Design review of the part built by this model. Coordinates are the model's own, in mm. Face numbers are marked on the shaded views. A direction names the side the tool comes from. Coordinates: 2 decimals unless noted, no trailing zeros. Write each loop counter-clockwise with the first axis right and the second up, starting at its lowest first coordinate (ties: lowest second). Pieces come first, ordered by that corner, then holes. Notation, with made-up numbers: (60.25, -37.5) -> (102.25, -37.5) arc R8 ccw to (102.25, -28.5) -> close; hole circle Ø7 at (39.25, 19.5). An arc over 180 degrees is marked (long way). Answer in a Markdown table with one row per item. Add a question column.
Item 1: To check wall thickness, follow line 1 (Z direction, x = -3.75, y = 8); line 2 (Z direction, x = -4.5, y = 9.5); line 3 (X direction, y = 94.5, z = -83.5). State the ranges of each line that lie inside material, in increasing order.
Item 2: Take a section at C-C, the plane z = -10. Write out the cut boundary in (x, y).
Item 3: For the marked faces 3, 4 and 5, list the 3-axis set-ups (+Z, -Z, +X, -X, +Y, -Y) from which the entire face can be reached by the end or side of a thin tool; tool diameter is ignored.
Item 4: Take a section at A-A, the plane x = -3.75. Write out the cut boundary in (y, z), and give its area (3 significant figures).
Item 5: Take a section at D-D, the plane z = -82.5. Write out the cut boundary in (x, y).
Item 6: Take a section at B-B, the plane y = 70. Write out the cut boundary in (x, z), and give its area (3 significant figures).
Item 7: Draft analysis for pull direction Z (two halves, no side actions). For the marked faces 1 and 2, state which applies: released by +Z, released by -Z, zero draft, split by the parting line, or undercut.
Item 8: Clearance check with flat-ended pins moving along their axes: P1, Ø1.4, axis at x = 0.5, y = 45.5, coming from the +Z side; P2, Ø4, axis at x = -0.5, z = -62, coming from the +Y side; P3, Ø1, axis at x = -2.5, y = 40, coming from the -Z side. State where each tip first meets the part, or that it passes through.
Autodesk Inventor part; units mm, degrees
ref_plane "YZ Plane" through (0, 0, 0) normal (1, 0, 0) x (0, 1, 0)
ref_plane "XZ Plane" through (0, 0, 0) normal (0, 1, 0) x (-1, 0, 0)
ref_plane "XY Plane" through (0, 0, 0) normal (0, 0, 1) x (1, 0, 0)
sketch "Sketch1" plane through (0, 0, 0) normal (0, 1, 0) x (-1, 0, 0)
  line L0 (0, 4.5) -> (0.254, 4.5)
  line L1 (0.254, -4.5) -> (0, -4.5)
  line L2 (6.35, 4.5) -> (6.35, -4.5)
  line L3 (6.35, 7.548) -> (6.35, 4.5)
  line L4 (6.35, -7.548) -> (6.35, -4.5)
  line L5 (0.254, 4.5) -> (6.35, 7.548)
  line L6 (0.254, -4.5) -> (6.35, -7.548)
  line L7 (0, 4.5) -> (0, -4.5)
  line L8 (0, -20.9) -> (0.254, -20.9)
  line L9 (0.254, -29.9) -> (0, -29.9)
  line L10 (6.35, -20.9) -> (6.35, -29.9)
  line L11 (6.35, -17.852) -> (6.35, -20.9)
  line L12 (6.35, -32.948) -> (6.35, -29.9)
  line L13 (0.254, -20.9) -> (6.35, -17.852)
  line L14 (0.254, -29.9) -> (6.35, -32.948)
  line L15 (0, -20.9) -> (0, -29.9)
  line L16 (0, -46.3) -> (0.254, -46.3)
  line L17 (0.254, -55.3) -> (0, -55.3)
  line L18 (6.35, -46.3) -> (6.35, -55.3)
  line L19 (6.35, -43.252) -> (6.35, -46.3)
  line L20 (6.35, -58.348) -> (6.35, -55.3)
  line L21 (0.254, -46.3) -> (6.35, -43.252)
  line L22 (0.254, -55.3) -> (6.35, -58.348)
  line L23 (0, -46.3) -> (0, -55.3)
  line L24 (0, -71.7) -> (0.254, -71.7)
  line L25 (0.254, -80.7) -> (0, -80.7)
  line L26 (6.35, -71.7) -> (6.35, -80.7)
  line L27 (6.35, -68.652) -> (6.35, -71.7)
  line L28 (6.35, -83.748) -> (6.35, -80.7)
  line L29 (0.254, -71.7) -> (6.35, -68.652)
  line L30 (0.254, -80.7) -> (6.35, -83.748)
  line L31 (0, -71.7) -> (0, -80.7)
  point P0 (0, 0)
  dimension "d16" = 6.096
  dimension "d25" = 9
  dimension "d26" = 3.048
  dimension "d27" = 3.048
  dimension "d28" = 0.254
  dimension "d29" = 0.254
  dimension "d33" = 25.4
extrude "Shape" add sketch "Sketch1" along normal blind 19.05 contours L0 L5 L3 L2 L4 L6 L1 L7 | L8 L13 L11 L10 L12 L14 L9 L15 | L16 L21 L19 L18 L20 L22 L17 L23
sketch "Sketch4" plane through (0, 0, 0) normal (0, -1, 0) x (1, 0, 0)
  line L0 (0, -55.3) -> (-0.254, -55.3) construction
  line L1 (0, -46.3) -> (0, -55.3) construction
  line L2 (-6.35, -43.252) -> (-0.254, -46.3) construction
  line L3 (-6.35, -58.348) -> (-6.35, -43.252) construction
  line L4 (-0.254, -55.3) -> (-6.35, -58.348) construction
  line L5 (-0.254, -46.3) -> (0, -46.3) construction
  line L6 (0, -93.6625) -> (-0.254, -93.6625)
  line L7 (-0.254, -93.6625) -> (-6.35, -90.6145)
  line L8 (-6.35, -105.7105) -> (-6.35, -90.6145)
  line L9 (-0.254, -55.3) -> (-6.35, -58.348)
  line L10 (-0.254, -102.6625) -> (-6.35, -105.7105)
  line L11 (0, -102.6625) -> (-0.254, -102.6625)
  line L12 (0, -102.6625) -> (0, -93.6625)
  line L13 (-0.254, -46.3) -> (0, -46.3)
  line L14 (0, -46.3) -> (0, -55.3)
  line L15 (0, -55.3) -> (0, -93.4) construction
  point P0 (0, 0)
  dimension "d43" = 38.1
extrude "Extrusion4" add sketch "Sketch4" against normal blind 100.2792
sketch "Sketch5" plane through (0, 0, -93.6625) normal (1, 0, 0) x (0, 0, -1)
  line L0 (12.048, 0) -> (12.048, 100.2792) construction
  line L1 (0, 100.2792) -> (9, 100.2792) construction
  line L2 (-101.2105, 0) -> (-101.2105, 19.05) construction
  line L3 (-86.1145, 0) -> (-101.2105, 0)
  line L4 (12.048, 0) -> (9, 0)
  line L5 (-101.2105, 0) -> (12.048, 0)
  line L6 (9, 100.2792) -> (12.048, 100.2792)
  line L7 (12.048, 0) -> (12.048, 100.2792)
  line L8 (12.048, 100.2792) -> (-13.352, 100.2792)
  line L9 (-13.352, 100.2792) -> (-13.352, 19.05)
  line L10 (-38.3625, 19.05) -> (-35.3145, 19.05)
  line L11 (-86.1145, 19.05) -> (-101.2105, 19.05)
  line L12 (-13.352, 19.05) -> (-101.2105, 19.05)
  line L13 (-101.2105, 19.05) -> (-101.2105, 0)
  point P0 (-93.6625, 0)
  point P1 (-101.2105, 100.2792)
  dimension "d46" = 25.4
extrude "Extrusion5" add sketch "Sketch5" along normal blind 1.27
sketch "Sketch6" plane through (-6.35, 0, -105.7105) normal (-1, 0, 0) x (0, 0, 1)
  line L0 (0, 100.2792) -> (15.096, 100.2792)
  line L1 (7.548, 100.2792) -> (7.548, 0) construction
  line L2 (113.2585, 0) -> (0, 0)
  circle A0 centre (7.548, 9.525) radius 1.9304
  circle A1 centre (7.548, 36.4744) radius 1.9304
  circle A2 centre (7.548, 63.4238) radius 1.9304
  circle A3 centre (7.548, 90.3732) radius 1.9304
  circle A4 centre (106.4852, 9.525) radius 1.9304
  circle A5 centre (79.5358, 9.525) radius 1.9304
  line L3 (113.2585, 0) -> (113.2585, 19.05)
  line L4 (25.4, 19.05) -> (113.2585, 19.05) construction
  line L5 (105.7105, 19.05) -> (105.7105, 0) construction
  line L6 (72.7625, 19.05) -> (87.8585, 19.05) construction
  line L7 (80.3105, 19.05) -> (80.3105, 0) construction
  line L8 (72.7625, 0) -> (87.8585, 0) construction
  line L9 (72.7625, 0) -> (72.7625, 19.05)
  line L10 (87.8585, 0) -> (87.8585, 19.05)
  dimension "d54" = 26.9494
  dimension "d48" = 3.8608
  dimension "d51" = 26.9494
  dimension "d57" = 3.8608
  dimension "d60" = 26.9494
  dimension "d69" = 0.7747
equation "\"d27\" = d26"
equation "\"d29\" = d28"
properties part number "Sliding test wall"
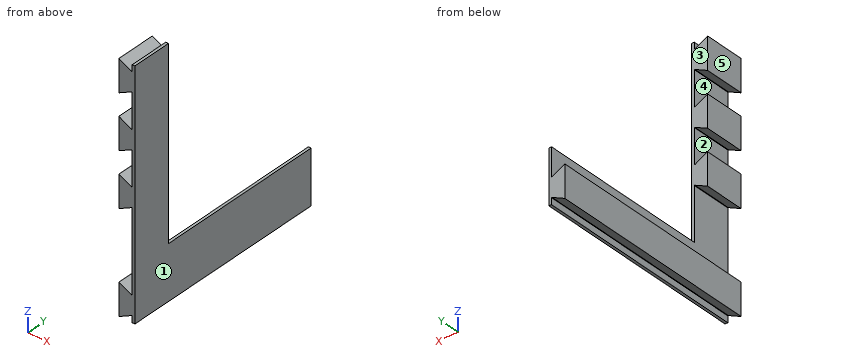
Answers:
| question | item | result |
|---|---|---|
| 1 | line 1 | z = -104.41 to -91.91, -57.05 to -44.55, -31.65 to -19.15, -6.25 to 6.25 |
| 1 | line 2 | z = -104.79 to -91.54, -57.42 to -44.18, -32.02 to -18.78, -6.62 to 6.62 |
| 1 | line 3 | x = 0 to 1.27 |
| 2 | outline | (0, 0) -> (1.27, 0) -> (1.27, 19.05) -> (0, 19.05) -> close |
| 3 | face 3 | +Z, +X, -X, +Y |
| 3 | face 4 | +Y, -Y |
| 3 | face 5 | +Z, -Z, -X, +Y, -Y |
| 4 | outline | (0, -104.41) -> (100.28, -104.41) -> (100.28, -91.91) -> (0, -91.91) -> close; (0, -57.05) -> (19.05, -57.05) -> (19.05, -44.55) -> (0, -44.55) -> close; (0, -31.65) -> (19.05, -31.65) -> (19.05, -19.15) -> (0, -19.15) -> close; (0, -6.25) -> (19.05, -6.25) -> (19.05, 6.25) -> (0, 6.25) -> close |
| 4 | area | 1,970 mm^2 |
| 5 | outline | (0, 0) -> (1.27, 0) -> (1.27, 100.28) -> (0, 100.28) -> close |
| 6 | outline | (-6.35, -105.71) -> (-0.25, -102.66) -> (0, -102.66) -> (0, -105.71) -> (1.27, -105.71) -> (1.27, -80.31) -> (0, -80.31) -> (0, -93.66) -> (-0.25, -93.66) -> (-6.35, -90.61) -> close |
| 6 | area | 108 mm^2 |
| 7 | face 1 | zero draft |
| 7 | face 2 | undercut |
| 8 | P1 | stops at z = -80.31 |
| 8 | P2 | stops at y = 19.05 |
| 8 | P3 | stops at z = -104.04 |
